Source: CAD feature listing. Evaluate the final solid. Frame: model axes, mm. Round coordinates to 2 decimals unless told otherwise and drop trailing zeros. Loops run counter-clockwise (first coordinate to the right, second up) from the corner with the lowest first, then second, coordinate; pieces in that order, holes last. Notation, with made-up numbers: (-36, 19.25) - (-14, 19.25) arc R10 ccw to (-14, 32.25) - close; hole circle Ø8 at (39.25, -27.75). An arc over 180 degrees is marked (long way). Write item = value, one per line. Start each with the question number.
from build123d import *

# Parameters (mm, degrees)
SKETCH1_R           = 4
SKETCH1_R_2         = 1.85
SKETCH1_R_3         = 2
SKETCH1_R_4         = 1.75
SKETCH1_W           = 14.5
SKETCH1_H           = 32
BOSS_EXTRUDE2_DEPTH = 6.35


with BuildPart() as part:
    # Sketch1 → Boss-Extrude2 (new body)
    with BuildSketch(Plane(origin=(0, 0, 0), x_dir=(0, 0, -1), z_dir=(1, 0, 0))):
        with BuildLine():
            Line((-16, 77.649446494), (-16, -13))
            ThreePointArc((-16, -13), (-14.535533906, -16.535533906), (-11, -18))
            Line((-11, -18), (119, -18))
            ThreePointArc((119, -18), (222.7396039, 64.546181173), (352, 94))
            ThreePointArc((352, 94), (363.313708499, 98.686291501), (368, 110))
            Line((368, 110), (368, 174))
            ThreePointArc((368, 174), (363.313708499, 185.313708499), (352, 190))
            ThreePointArc((352, 190), (180.885272405, 173.600745723), (16, 125))
            ThreePointArc((16, 125), (-7.249835994, 106.224238345), (-16, 77.649446494))
        make_face()
        with Locations((352, 110)):
            Circle(SKETCH1_R, mode=Mode.SUBTRACT)
        with Locations((352, 118)):
            Circle(SKETCH1_R_2, mode=Mode.SUBTRACT)
        with Locations((352, 126)):
            Circle(SKETCH1_R, mode=Mode.SUBTRACT)
        with Locations((352, 134)):
            Circle(SKETCH1_R_2, mode=Mode.SUBTRACT)
        with Locations((352, 142)):
            Circle(SKETCH1_R, mode=Mode.SUBTRACT)
        with Locations((360, 110)):
            Circle(SKETCH1_R_2, mode=Mode.SUBTRACT)
        with Locations((352, 102)):
            Circle(SKETCH1_R_2, mode=Mode.SUBTRACT)
        with Locations((344, 110)):
            Circle(SKETCH1_R_2, mode=Mode.SUBTRACT)
        with Locations((346.343145751, 136.343145751)):
            Circle(SKETCH1_R_2, mode=Mode.SUBTRACT)
        with Locations((344, 142)):
            Circle(SKETCH1_R_2, mode=Mode.SUBTRACT)
        with Locations((346.343145751, 147.656854249)):
            Circle(SKETCH1_R_2, mode=Mode.SUBTRACT)
        with Locations((352, 150)):
            Circle(SKETCH1_R_2, mode=Mode.SUBTRACT)
        with Locations((357.656854249, 147.656854249)):
            Circle(SKETCH1_R_2, mode=Mode.SUBTRACT)
        with Locations((360, 142)):
            Circle(SKETCH1_R_2, mode=Mode.SUBTRACT)
        with Locations((357.656854249, 136.343145751)):
            Circle(SKETCH1_R_2, mode=Mode.SUBTRACT)
        with Locations((344, 174)):
            Circle(SKETCH1_R_2, mode=Mode.SUBTRACT)
        with Locations((352, 182)):
            Circle(SKETCH1_R_2, mode=Mode.SUBTRACT)
        with Locations((360, 174)):
            Circle(SKETCH1_R_2, mode=Mode.SUBTRACT)
        with Locations((352, 158)):
            Circle(SKETCH1_R, mode=Mode.SUBTRACT)
        with Locations((352, 166)):
            Circle(SKETCH1_R_2, mode=Mode.SUBTRACT)
        with Locations((352, 174)):
            Circle(SKETCH1_R, mode=Mode.SUBTRACT)
        Circle(SKETCH1_R, mode=Mode.SUBTRACT)
        with Locations((8, 0)):
            Circle(SKETCH1_R_2, mode=Mode.SUBTRACT)
        with Locations((0, -8)):
            Circle(SKETCH1_R_2, mode=Mode.SUBTRACT)
        with Locations((-8, 0)):
            Circle(SKETCH1_R_2, mode=Mode.SUBTRACT)
        with Locations((0, 8)):
            Circle(SKETCH1_R_2, mode=Mode.SUBTRACT)
        with Locations((150, 28.62526107)):
            Circle(SKETCH1_R_3, mode=Mode.SUBTRACT)
        with Locations((150, 44.62526107)):
            Circle(SKETCH1_R_3, mode=Mode.SUBTRACT)
        with Locations((150, 60.62526107)):
            Circle(SKETCH1_R_3, mode=Mode.SUBTRACT)
        with Locations((243, 168.269053261)):
            Circle(SKETCH1_R, mode=Mode.SUBTRACT)
        with Locations((251, 168.269053261)):
            Circle(SKETCH1_R_2, mode=Mode.SUBTRACT)
        with Locations((243, 160.269053261)):
            Circle(SKETCH1_R_2, mode=Mode.SUBTRACT)
        with Locations((235, 168.269053261)):
            Circle(SKETCH1_R_2, mode=Mode.SUBTRACT)
        with Locations((243, 176.269053261)):
            Circle(SKETCH1_R_2, mode=Mode.SUBTRACT)
        with Locations((23.5, 117.5)):
            Circle(SKETCH1_R_4, mode=Mode.SUBTRACT)
        with Locations((111.5, 117.5)):
            Circle(SKETCH1_R_4, mode=Mode.SUBTRACT)
        with Locations((111.5, -10.5)):
            Circle(SKETCH1_R_4, mode=Mode.SUBTRACT)
        with Locations((23.5, -10.5)):
            Circle(SKETCH1_R_4, mode=Mode.SUBTRACT)
        with Locations((136.25, 44.62526107)):
            Rectangle(SKETCH1_W, SKETCH1_H, mode=Mode.SUBTRACT)
    extrude(amount=BOSS_EXTRUDE2_DEPTH)


solid = part.part
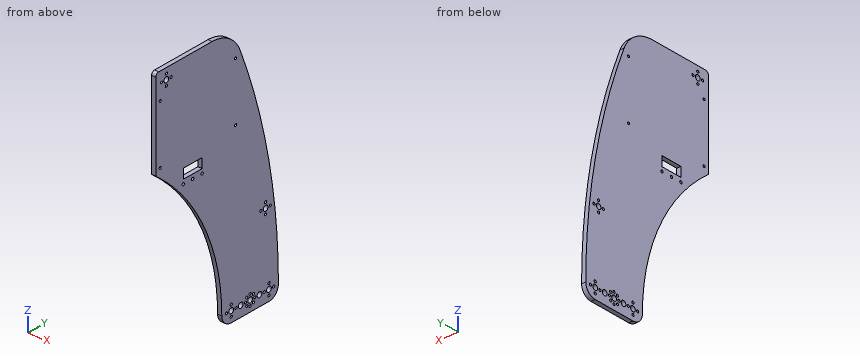
(1) Cut plane B-B (z = -319.5). Output: boundary loops of the cut face in (x, y), and give its area (3 significant figures).
(2) Pin query (flat end, axial travel): P1, Ø2, axis at x = 3, z = -156, coming from the +Y side; P2, Ø3, axis at x = 2, y = 108.5, coming from the -Z side; P3, Ø3, axis at x = 4, z = -203, coming from the +Y side; P4, Ø3, axis at x = 1.5, z = -227.5, coming from the -Y side. Return the tip coordinate at first contact, or that it passes through.
(3) Cut plane A-A (x = 5.25). State how many separate pieces and enclosed holes the cut face has, and give its area (3 significant figures).
(4) Material intervals for line 1 along Y through (x, z) = (5, -360); line 2 along Y through (x, z) = (3, -235); line 3 along Y through (x, z) = (4.5, 0), sorted ascending. Write a range as from..to.
(5) Cut plane C-C (y = 84.5). Output: boundary loops of the cut face in (x, z).
Solution:
q1.outline = (0, 92.22) - (6.35, 92.22) - (6.35, 189.41) - (0, 189.41) - close
q1.area = 617 mm^2
q2.P1 = 168.64
q2.P2 = -368
q2.P3 = 177.84
q2.P4 = 66.09
q3.separate_pieces = 1
q3.enclosed_holes = 39
q3.area = 49,000 mm^2
q4.line_1 = 96.14..108.15, 111.85..140.15, 143.85..172.15, 175.85..187.86
q4.line_2 = 70.1..166.42, 170.12..182.37
q4.line_3 = -18..-9.85, -6.15..-4, 4..6.15, 9.85..114.76
q5.outline = (0, -277.31) - (6.35, -277.31) - (6.35, 15.54) - (0, 15.54) - close
